CAD build for the part. Positions are in the model's coordinates, mm. Face numbers are marked on the shaded views. Give positions to 0.01 mm unless a question says otherwise; leave off trailing zeros. Loops run counter-clockwise (first coordinate to the right, second up) from the corner with the lowest first, then second, coordinate; pieces in that order, holes last.
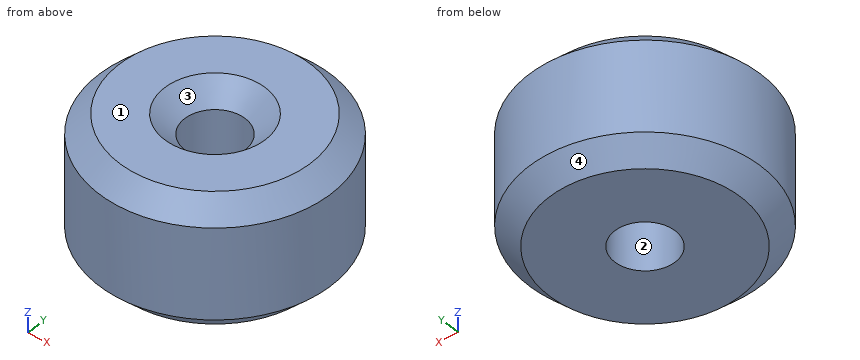
```python
from build123d import *

# Parameters (mm, degrees)
F0_R     = 11.5
F0_R_2   = 3
F1_DEPTH = 13
F2_SIZE  = 2
F3_SIZE  = 2
F4_SIZE  = 2


with BuildPart() as f1:
    # F0 (on Top) → F1 (new body)
    with BuildSketch(Plane.XY):
        with Locations((-42.798914, 37.472825)):
            Circle(F0_R)
        with Locations((-42.798914, 37.472825)):
            Circle(F0_R_2, mode=Mode.SUBTRACT)
    extrude(amount=F1_DEPTH)

    # F2
    f2_edges = [f1.edges().sort_by_distance(p)[0] for p in [
        (-54.298914, 37.472825, 13),
    ]]
    chamfer(f2_edges, length=F2_SIZE)

    # F3
    f3_edges = [f1.edges().sort_by_distance(p)[0] for p in [
        (-54.298914, 37.472825, 0),
    ]]
    chamfer(f3_edges, length=F3_SIZE)

    # F4
    f4_edges = [f1.edges().sort_by_distance(p)[0] for p in [
        (-45.798914, 37.472825, 13),
    ]]
    chamfer(f4_edges, length=F4_SIZE)


solid = f1.part
```
1. Saw through at A-A, the plane z = 1. List the corners of the cut face in (x, y).
Responses:
outline: circle Ø21 at (-42.8, 37.47); hole circle Ø6 at (-42.8, 37.47)
2. Drop flat-ended pins along their axis: pin 1 (2 mm diameter, centred on y = 40, z = 6.5, fed in from +X); pin 2 (2 mm diameter, centred on y = 43.5, z = 4, fed in from -X); pin 3 (4 mm diameter, centred on x = -48.5, z = 11.5, fed in from +Y). Give the stop position or say it passes through.
Responses:
pin 1: stops at x = -31.4
pin 2: stops at x = -53.14
pin 3: stops at y = 48.34
3. Pull direction Y, two halves, no side cores. Call the marked faces 1, 2, 3 and 4: released by +Y, released by -Y, zero draft, split by the parting line, or undercut.
Responses:
face 1: zero draft
face 2: undercut
face 3: undercut
face 4: split by the parting line
4. Probe line 1 along Y through (x, z) = (-41.25, 2.75); line 2 along Y through (x, z) = (-45, 2.5); line 3 along X through (y, z) = (31, 5.5). List the from-to ranges inside material, lowest first.
Responses:
line 1: y = 26.08 to 34.9, 40.04 to 48.87
line 2: y = 26.19 to 35.43, 39.51 to 48.76
line 3: x = -52.3 to -33.29
5. Saw through at B-B, the plane z = 12.25. List the corners of the cut face in (x, y).
Responses:
outline: circle Ø20.5 at (-42.8, 37.47); hole circle Ø8.5 at (-42.8, 37.47)
